Design review of the part built by this model. Coordinates are the model's own, in mm. Coordinates: 2 decimals unless noted, no trailing zeros. Write each loop counter-clockwise with the first axis right and the second up, starting at its lowest first coordinate (ties: lowest second). Pieces come first, ordered by that corner, then holes. Notation, with made-up numbers: (73, -23.75) - (95, -23.75) arc R8 ccw to (95, -14.75) - close; hole circle Ø11 at (50.5, -24.5). An arc over 180 degrees is marked (long way). Answer as CSV lines item,"result". Start each with the question number.
Q1. Clearance check with flat-ended pins moving along their axes: pin 1 (1.5 mm diameter, centred on x = 20, y = 3.5, fed in from -Z); pin 2 (2.5 mm diameter, centred on x = 6.32, y = 48.82, fed in from -Z); pin 3 (6 mm diameter, centred on y = 26.5, z = 1.5, fed in from -X); pin 4 (4.5 mm diameter, centred on x = 121.5, y = -25, fed in from -Z). State where each tip first meets the part, or that it passes through.
Q2. We need section C-C (y = -2). Write out the cut boundary in (x, z), plus the area to 3 significant figures.
Q3. We need section D-D (y = 27.5). Write out the cut boundary in (x, z), plus the area to 3 significant figures.
Q4. For line 1 along X through (y, z) = (48.55, 1.8); line 2 along X through (y, z) = (37, 1.75); line 3 along Z through (x, y) = (115.5, -1.2), list the stretches that pass through material, from the lowest coordinate up. Write a range as [from, to].
Q5. We need section B-B (x = 26). Write out the cut boundary in (y, z).
Q6. We need section A-A (y = -26). Write out the cut boundary in (x, z), plus the area to 3 significant figures.
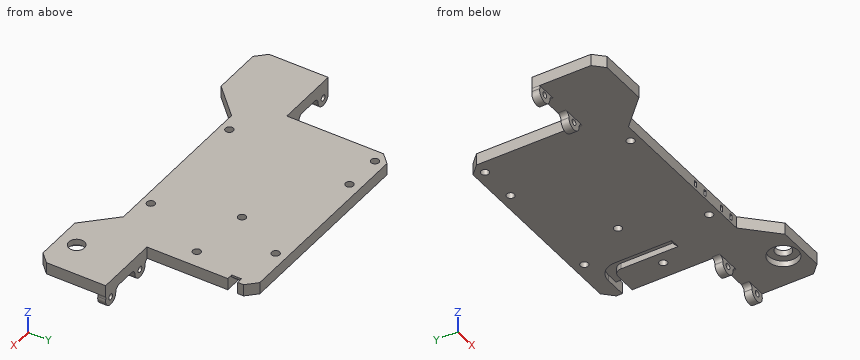
Autodesk Inventor part; units mm, degrees
ref_plane "Work Plane1" through (55, 0, 6) normal (1, 0, 0) x (0, 0, -1)
ref_plane "YZ Plane" through (0, 0, 0) normal (1, 0, 0) x (0, 1, 0)
ref_plane "XZ Plane" through (0, 0, 0) normal (0, 1, 0) x (-1, 0, 0)
sketch "Sketch1" plane through (0, 0, 0) normal (0, 0, 1) x (1, 0, 0)
  line L0 (-32.5, 0) -> (0, 0)
  line L1 (0, 0) -> (0, 54.05)
  line L2 (0, 54.05) -> (110, 54.05)
  line L3 (110, 54.05) -> (110, 0)
  line L4 (110, 0) -> (142.5, 0)
  line L5 (142.5, 0) -> (142.5, -35)
  line L6 (142.5, -35) -> (112.5, -35)
  line L7 (112.5, -35) -> (97.5, -20)
  line L8 (97.5, -20) -> (12.5, -20)
  line L9 (12.5, -20) -> (-2.5, -35)
  line L10 (-2.5, -35) -> (-32.5, -35)
  line L11 (-32.5, -35) -> (-32.5, 0)
  dimension "d0" = 135
  dimension "d1" = 135
  dimension "d2" = 110
  dimension "d3" = 54.05
  dimension "d4" = 35
  dimension "d5" = 32.5
  dimension "d6" = 20
  dimension "d7" = 30
extrude "Extrusion1" add sketch "Sketch1" along normal blind 6
chamfer "Chamfer1" distance 5 angle 45 4 edges at (0, 54.05, 3) (110, 54.05, 3) (-32.5, -35, 3) (142.5, -35, 3)
sketch "Sketch2" plane through (110, 0, 0) normal (0, 1, 0) x (1, 0, 0)
  circle A0 centre (-138.5, 2.5) radius 1.5
  circle A1 centre (-115.5, 2.5) radius 1.5
  line L0 (-142.5, 0) -> (-142.5, -6)
  line L1 (-110, 0) -> (-142.5, 0)
  circle A2 centre (-138.5, 2.5) radius 4
  line L2 (-142.5, 0) -> (-112.5, 0)
  arc A3 (-142.5, 0) -> (-142.3846, 1.5461) centre (-144.8125, 0.95) ccw
  arc A4 (-134.5, 2.5) -> (-132, 0) centre (-132, 2.5) ccw
  arc A5 (-122, 0) -> (-119.5, 2.5) centre (-122, 2.5) ccw
  arc A6 (-111.5, 2.5) -> (-109, 0) centre (-109, 2.5) ccw
  circle A7 centre (-115.5, 2.5) radius 4
  line L3 (-109, 0) -> (-112.3775, 0)
  line L4 (-112.5, 0) -> (-97.5, 0)
  point P0 (-122, 0)
  point P1 (-132, 0)
  point P2 (-118.6225, 0)
  point P3 (-112.3775, 0)
  dimension "d13" = 3
  dimension "d14" = 3
  dimension "d15" = 4
  dimension "d16" = 27
  dimension "d17" = 2.5
  dimension "d18" = 8
extrude "Extrusion2" add sketch "Sketch2" against normal blind 4 contours L1 A2 A4 | L1 A7 A6 L3 | L1 A7 | L1 A5 A7 | L1 A2 | L1 A3 A2 picked at (-115.6011, 0.337) picked at (-138.4397, 0.337)
sketch "Sketch3" plane through (0, 0, 0) normal (0, 0, -1) x (-1, 0, 0)
  line L0 (-105, 54.05) -> (-5, 54.05)
  line L1 (0, 49.05) -> (0, 0)
  line L2 (-110, 0) -> (-110, 49.05)
  point P0 (-84, 48.55)
  point P1 (-26, 48.55)
  dimension "d21" = 5.5
  dimension "d22" = 26
  dimension "d23" = 26
hole "Hole1" at (84, 48.55, 0) at (26, 48.55, 0) direction (0, 0, 1) diameter 4 depth 24
sketch "Sketch4" plane through (12.5, -20, 0) normal (0, -1, 0) x (1, 0, 0)
  line L0 (74, 1.5) -> (72.5, 1.5)
  line L1 (72.5, 1.5) -> (72.5, 4.5)
  line L2 (72.5, 4.5) -> (74, 4.5)
  line L3 (74, 4.5) -> (74, 1.5)
  line L4 (77, 1.5) -> (77, 4.5)
  line L5 (-15, 0) -> (-15, 6)
  line L6 (85, 0) -> (85, 6)
  line L7 (53.5, 1.5) -> (52, 1.5)
  line L8 (52, 1.5) -> (52, 4.5)
  line L9 (52, 4.5) -> (53.5, 4.5)
  line L10 (53.5, 4.5) -> (53.5, 1.5)
  line L11 (56.5, 1.5) -> (56.5, 4.5)
  point P0 (-12.5, 0)
  point P1 (72.5, 3)
  point P2 (-15, 3)
  point P3 (77, 3)
  point P4 (74, 3)
  point P5 (53.5, 3)
  point P6 (56.5, 3)
  dimension "d31" = 1.5
  dimension "d32" = 3
  dimension "d33" = 3
  dimension "d35" = 8
  dimension "d36" = 1.5
  dimension "d37" = 3
  dimension "d38" = 3
  dimension "d39" = 16
revolve "Revolution1" cut sketch "Sketch4" angle 360 about axis through (89.5, -20, 1.5) along (0, 0, 1) contours L0 L1 L2 L3
revolve "Revolution2" cut sketch "Sketch4" angle 360 about axis through (69, -20, 1.5) along (0, 0, 1) contours L7 L8 L9 L10
ref_plane "Work Plane1" through (55, 0, 6) normal (1, 0, 0) x (0, 0, -1)
mirror "Mirror1" about plane through (55, 0, 6) normal (1, 0, 0) of "Extrusion2"
sketch "Sketch5" plane through (0, 0, 6) normal (0, 0, 1) x (1, 0, 0)
  circle A0 centre (101.2237, 19.6209) radius 1.6
  circle A1 centre (70.2706, 22.6087) radius 1.6
  circle A2 centre (21.34, -15.4078) radius 1.6
  circle A3 centre (83.2562, -15.291) radius 1.6
  circle A4 centre (6.3179, 48.8175) radius 1.6
  circle A5 centre (70.2706, 22.6087) radius 4
  circle A6 centre (101.2237, 19.6209) radius 4
  circle A7 centre (83.2562, -15.291) radius 4
  circle A8 centre (21.34, -15.4078) radius 4
  circle A9 centre (6.3179, 48.8175) radius 4
  line L0 (109, 0) -> (109, -4)
  line L1 (12.5, -20) -> (97.5, -20)
  line L2 (110, 0) -> (97.5, -20)
  circle A10 centre (26, 48.55) radius 2
  circle A11 centre (84, 48.55) radius 2
  circle A12 centre (26, 48.55) radius 4
  circle A13 centre (84, 48.55) radius 4
  circle A14 centre (84, 48.55) radius 2
  circle A15 centre (26, 48.55) radius 2
  line L3 (105, 54.05) -> (110, 49.05)
  line L4 (105, 54.05) -> (5, 54.05)
  line L5 (0, 49.05) -> (5, 54.05)
  line L6 (0, 49.05) -> (0, 0)
  line L7 (0, 0) -> (-32.5, 0)
  line L8 (-32.5, 0) -> (-32.5, -30)
  line L9 (-27.5, -35) -> (-2.5, -35)
  line L10 (-2.5, -35) -> (12.5, -20)
  line L11 (12.5, -20) -> (97.5, -20)
  line L12 (97.5, -20) -> (112.5, -35)
  line L13 (112.5, -35) -> (137.5, -35)
  line L14 (142.5, -30) -> (142.5, 0)
  line L15 (142.5, 0) -> (110, 0)
  line L16 (110, 0) -> (110, 49.05)
  line L17 (0, 49.05) -> (5, 54.05)
  line L18 (105, 54.05) -> (5, 54.05)
  line L19 (105, 54.05) -> (110, 49.05)
  line L20 (142.5, -30) -> (137.5, -35)
  line L21 (-27.5, -35) -> (-32.5, -30)
  circle A16 centre (6.3179, 48.8175) radius 1.6
  circle A17 centre (21.34, -15.4078) radius 1.6
  circle A18 centre (70.2706, 22.6087) radius 1.6
  circle A19 centre (101.2237, 19.6209) radius 1.6
  circle A20 centre (83.2562, -15.291) radius 1.6
  line L22 (110, 0) -> (110, 49.05)
  line L23 (0, 49.05) -> (0, 0)
  dimension "d41" = 8
  dimension "d82" = 5.5
  dimension "d83" = 5.5
  dimension "d84" = 26
  dimension "d85" = 26
hole "Hole2" at (6.3179, 48.8175, 6) at (70.2706, 22.6087, 6) at (101.2237, 19.6209, 6) at (83.2562, -15.291, 6) at (21.34, -15.4078, 6) direction (0, 0, -1) diameter 4 depth 24
sketch "Sketch6" plane through (0, 0, 0) normal (0, 0, -1) x (-1, 0, 0)
  line L0 (-110, 0) -> (-110, 49.05)
  line L1 (-110, 46.05) -> (-107, 46.05)
  line L2 (-107, 46.05) -> (-90, 46.05)
  line L3 (-90, 46.05) -> (-90, 10)
  line L4 (-90, 10) -> (-95, 10)
  line L5 (-95, 10) -> (-95, 41.05)
  line L6 (-95, 41.05) -> (-110, 41.05)
  line L7 (-110, 0) -> (-110, 49.05)
  line L8 (-12.5, -20) -> (-97.5, -20)
  line L9 (-107, 46.05) -> (-107, 41.05)
  point P0 (0, 0)
  dimension "d49" = 30
  dimension "d50" = 5
  dimension "d51" = 5
  dimension "d55" = 15
  dimension "d68" = 3
  dimension "d69" = 3
extrude "Extrusion3" cut sketch "Sketch6" against normal blind 3
extrude "Extrusion4" cut sketch "Sketch6" against normal through all contours L0 L1 L9 L6
fillet "Fillet1" radius 4 1 edges at (95, 41.05, 1.5)
fillet "Fillet2" radius 9 1 edges at (90, 46.05, 1.5)
chamfer "Chamfer2" distance 2 angle 45 2 edges at (92.5, 10, 0) (107, 43.55, 3)
sketch "Sketch7" plane through (0, 0, 0) normal (0, 0, -1) x (-1, 0, 0)
  circle A0 centre (-125, -26) radius 4
  circle A1 centre (-125, -26) radius 5 construction
  circle A2 centre (-125, -26) radius 9 construction
  line L0 (-112.5, -35) -> (-137.5, -35)
  circle A3 centre (-125, -26) radius 7.5
  point P0 (0, 0)
  point P1 (-125, -35)
  dimension "d70" = 8
  dimension "d71" = 10
  dimension "d72" = 18
  dimension "d75" = 15
extrude "Extrusion5" cut sketch "Sketch7" against normal through all contours A0
extrude "Extrusion6" cut sketch "Sketch7" against normal blind 3 contours A0 | A3
equation "\"d51\" = d50"
equation "\"d61\" = d60 + d50"
equation "\"MotorHeight\" = MotorHeightBase"
properties part number "Driver Board Mount"
Results list:
1,pin 1,"stops at z = 0"
1,pin 2,"passes through"
1,pin 3,"stops at x = 0"
1,pin 4,"stops at z = 3"
2,outline,"(-32.5, 0) arc R2.5 cw to (-32.38, -1.55) arc R4 ccw (long way) to (-24.5, -2.5) arc R2.5 cw to (-22, 0) - (-12, 0) arc R2.5 cw to (-9.5, -2.5) arc R4 ccw to (-1.5, -2.5) arc R2.5 cw to (1, 0) - (109, 0) arc R2.5 cw to (111.5, -2.5) arc R4 ccw to (119.5, -2.5) arc R2.5 cw to (122, 0) - (132, 0) arc R2.5 cw to (134.5, -2.5) arc R4 ccw (long way) to (142.38, -1.55) arc R2.5 cw to (142.5, 0) - (142.5, 6) - (-32.5, 6) - close; hole circle Ø3 at (-28.5, -2.5); hole circle Ø3 at (-5.5, -2.5); hole circle Ø3 at (115.5, -2.5); hole circle Ø3 at (138.5, -2.5)"
2,area,"1,210 mm2"
3,outline,"(0, 0) - (90, 0) - (90, 3) - (95, 3) - (95, 0) - (110, 0) - (110, 6) - (0, 6) - close"
3,area,"645 mm2"
4,line 1,"x = [0, 4.34], [8.3, 24], [28, 82], [86, 110]"
4,line 2,"x = [0, 90], [95, 110]"
4,line 3,"z = [-6.5, -4], [-1, 6]"
5,outline,"(-20, 0) - (46.55, 0) - (46.55, 6) - (-20, 6) - close; (50.55, 0) - (54.05, 0) - (54.05, 6) - (50.55, 6) - close"
6,outline,"(-32.5, 0) - (6.5, 0) - (6.5, 6) - (-32.5, 6) - close; (103.5, 0) - (117.5, 0) - (117.5, 3) - (121, 3) - (121, 6) - (103.5, 6) - close; (129, 3) - (132.5, 3) - (132.5, 0) - (142.5, 0) - (142.5, 6) - (129, 6) - close"
6,area,"399 mm2"
